Autodesk Inventor part; units mm, degrees
ref_plane "Work Plane1" through (34, 0, 0) normal (1, 0, 0) x (0, 0, -1)
ref_plane "YZ Plane" through (0, 0, 0) normal (1, 0, 0) x (0, 1, 0)
ref_plane "XZ Plane" through (0, 0, 0) normal (0, 1, 0) x (-1, 0, 0)
sketch "Sketch1" plane through (0, 0, 0) normal (1, 0, 0) x (0, 1, 0)
  line L0 (0, 0) -> (4, 0)
  line L1 (4, 6) -> (4, 130)
  line L2 (4, 130) -> (0, 130)
  line L3 (0, 130) -> (0, 0)
  line L4 (10, 0) -> (74, 0)
  line L5 (74, 0) -> (74, -4)
  line L6 (74, -4) -> (10, -4)
  line L7 (0, 6) -> (0, 0)
  line L8 (4, 45) -> (49, 0)
  arc A0 (4, 6) -> (10, 0) centre (10, 6) ccw
  arc A1 (0, 6) -> (10, -4) centre (10, 6) ccw
  line L9 (4, 6) -> (10, 0)
  point P0 (0, -4)
  point P1 (0, 6)
  point P2 (2, 0)
  dimension "d0" = 4
  dimension "d1" = 130
  dimension "d2" = 70
  dimension "d3" = 45
  dimension "d4" = 45
  dimension "d35" = 10
extrude "Extrusion1" add sketch "Sketch1" along normal blind 68 contours A1 L3 L2 L1 A0 L4 L5 L6
extrude "Extrusion2" add sketch "Sketch1" along normal blind 4 contours L8 L4 L9 L1
extrude "Extrusion3" add sketch "Sketch1" against normal blind 4 from surface at 68 contours L8 L4 L9 L1
sketch "Sketch2" plane through (0, 74, 0) normal (0, 0, 1) x (1, 0, 0)
  line L0 (0, 0) -> (68, 0) construction
  line L1 (4, 0) -> (64, 0) construction
  line L2 (64, 0) -> (64, -60) construction
  line L3 (64, -60) -> (4, -60) construction
  line L4 (4, -60) -> (4, 0) construction
  line L5 (4, -25) -> (4, -70) construction
  line L6 (64, -70) -> (64, -25) construction
  line L7 (10.43, -6.43) -> (57.57, -6.43) construction
  line L8 (57.57, -6.43) -> (57.57, -53.57) construction
  line L9 (57.57, -53.57) -> (10.43, -53.57) construction
  line L10 (10.43, -53.57) -> (10.43, -6.43) construction
  line L11 (4, 0) -> (64, -60) construction
  line L12 (4, -60) -> (64, 0) construction
  circle A0 centre (34, -30) radius 20
  circle A1 centre (10.43, -6.43) radius 2.5
  circle A2 centre (57.57, -6.43) radius 2.5
  circle A3 centre (57.57, -53.57) radius 2.5
  circle A4 centre (10.43, -53.57) radius 2.5
  dimension "d26" = 60
  dimension "d27" = 60
  dimension "d28" = 47.14
  dimension "d29" = 40
  dimension "d30" = 5
extrude "Extrusion4" cut sketch "Sketch2" against normal through all
chamfer "Chamfer1" distance 6 angle 45 4 edges at (68, 74, -2) (0, 74, -2) (68, 2, 130) (0, 2, 130)
ref_plane "Work Plane1" through (34, 0, 0) normal (1, 0, 0) x (0, 0, -1)
properties part number "MotorBracket" material "Stainless Steel"
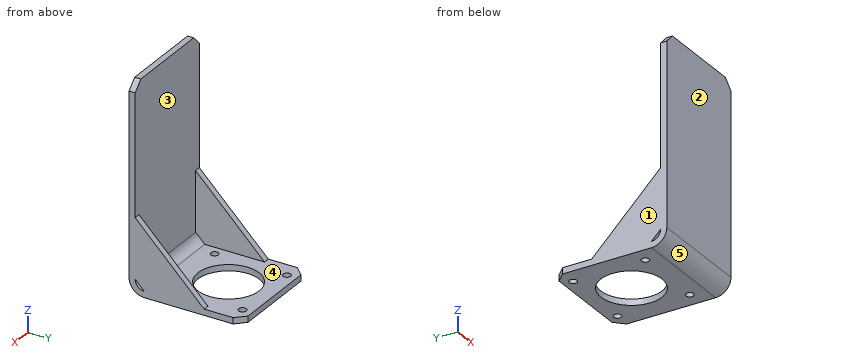
Verification items for the finished model (mm, model axes). Face numbers are marked on the shaded views. A direction names the side the tool comes from. Round coordinates to 2 decimals unless told otherwise and drop trailing zeros. Write each loop counter-clockwise with the first axis right and the second up, starting at its lowest first coordinate (ties: lowest second). Pieces come first, ordered by that corner, then holes.
1. Section check A-A on x = 34. Enter the section's corners in (y, z), plus the area to 3 significant figures.
2. Draft check along Y on the marked faces 1, 2 and 3. Enter one of: +Y half, -Y half, draft (parallel to the pull), parting line (faces both ways), or undercut.
3. Scan lines: L1, parallel to Y at x = 57.57, z = -1.8; L2, parallel to Y at x = 57.57, z = -2.45; L3, parallel to X at y = 67, z = -1. Record each from-to range of solid material in increasing order.
4. Access from +Z, -Z, +X, -X, +Y, -Y to the whole of each face (thin tool, end or side, straight path). Record for the marked faces 4 and 5.
5. Section check C-C on y = 12. Enter the section's corners in (x, z), plus the area to 3 significant figures.
6. Section check B-B on x = 57.57. Enter the section's corners in (y, z), plus the area to 3 significant figures.
7. Section check D-D on z = 12. Enter the section's corners in (x, y).
8. Gauge pin test, flat ends, axial feed: P1, Ø5, axis at x = 52, z = 44, coming from the +Y side; P2, Ø8, axis at x = 10.43, y = 67.57, coming from the +Z side; P3, Ø3, axis at x = 57.57, y = 67.57, coming from the +Z side. Record the tip position at first contact, or that the pin passes through.
Answer:
1. outline: (0, 6) arc R10 ccw to (10, -4) - (24, -4) - (24, 0) - (10, 0) arc R6 cw to (4, 6) - (4, 130) - (0, 130) - close; (64, -4) - (74, -4) - (74, 0) - (64, 0) - close
1. area: 642 mm2
2. face 1: draft
2. face 2: -Y half
2. face 3: +Y half
3. L1: y = 3.74 to 17.93, 22.93 to 65.07, 70.07 to 74
3. L2: y = 4.65 to 17.93, 22.93 to 65.07, 70.07 to 74
3. L3: x = 0 to 8, 12.86 to 55.14, 60 to 68
4. face 4: +Z, +Y
4. face 5: -Z, +X, -X, -Y
5. outline: (0, -4) - (68, -4) - (68, 37) - (64, 37) - (64, 0) - (4, 0) - (4, 37) - (0, 37) - close
5. area: 568 mm2
6. outline: (0, 6) arc R10 ccw to (10, -4) - (17.93, -4) - (17.93, 0) - (10, 0) arc R6 cw to (4, 6) - (4, 130) - (0, 130) - close; (22.93, -4) - (65.07, -4) - (65.07, 0) - (22.93, 0) - close; (70.07, -4) - (74, -4) - (74, 0) - (70.07, 0) - close
6. area: 762 mm2
7. outline: (0, 0) - (68, 0) - (68, 37) - (64, 37) - (64, 4) - (4, 4) - (4, 37) - (0, 37) - close
8. P1: stops at y = 4
8. P2: stops at z = 0
8. P3: passes through
